Part print with two shaded views. Sizes in mm from the minimum x, y, z corner. A direction names the side the tool comes from. Coordinates: 2 decimals unless noted, no trailing zeros. Loops run counter-clockwise (first coordinate to the right, second up) from the corner with the lowest first, then second, coordinate; pieces in that order, holes last. Notation, with made-up numbers: (31.25, -35) -> (70.25, -35) arc R12 ccw to (70.25, -15) -> close; hole circle Ø8 at (64.25, 37.5). An arc over 180 degrees is marked (long way). Write each question's results on one line, items separated by ' | '.
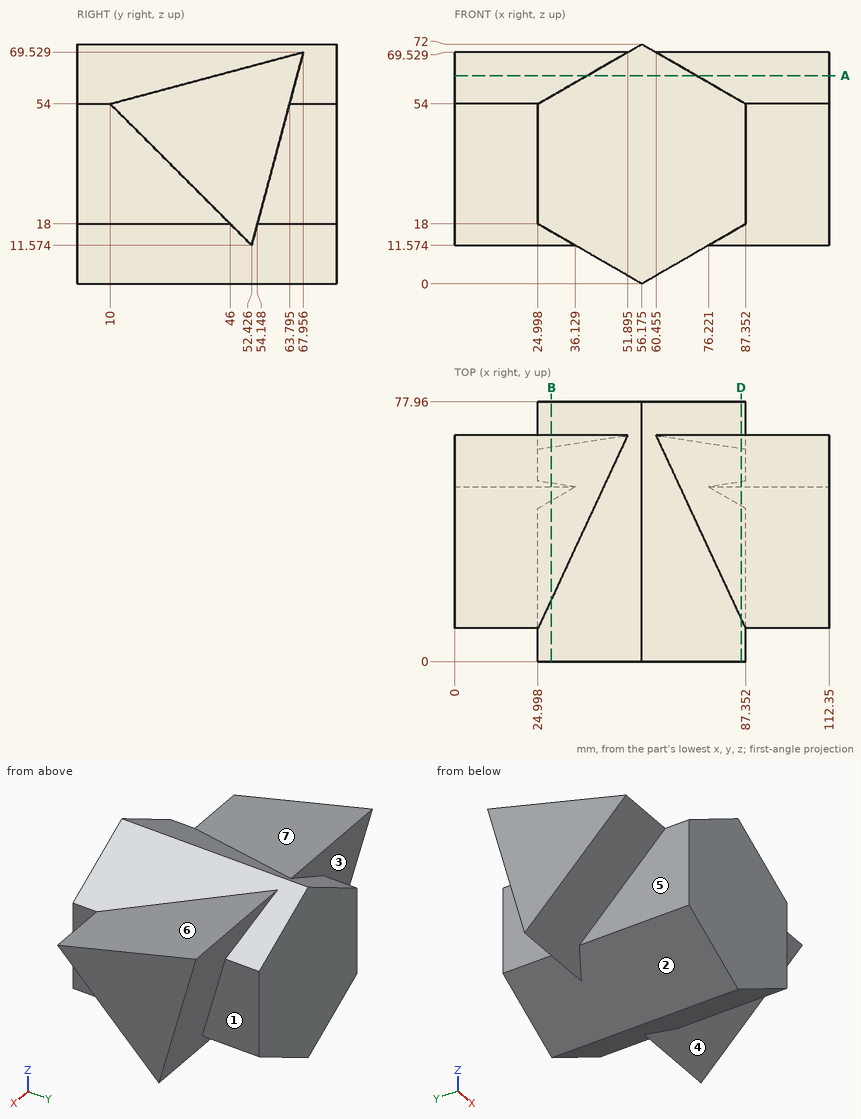
Q1. Pull direction X, two halves, no side cores. Call the marked faces 1, 2 and 3: +X half, -X half, draft (parallel to the pull), parting line (faces both ways), or undercut.
Results are:
face 1: +X half | face 2: -X half | face 3: draft
Q2. Which spindle directions (+Z, -Z, +X, -X, +Y, -Y) get a long thin tool onto all of the face, cutting with end or side? Do the marked faces 4, 5, 6 and 7. Say none if no direction does.
Results are:
face 4: -Z, +X, -Y | face 5: -Z, -X, -Y | face 6: +Z, +X, -Y | face 7: +Z, -X, -Y
Q3. Drop flat-ended pins along their axis: pin 1 (1.5 mm diameter, centred on x = 17.5, z = 31.5, fed in from -Y); pin 2 (1.5 mm diameter, centred on x = 17, y = 31.5, fed in from -Z); pin 3 (1.5 mm diameter, centred on x = 85, y = 28.5, fed in from -Z); pin 4 (1.5 mm diameter, centred on y = 46.5, z = 32.5, fed in from -X). Give the stop position or say it passes through.
Results are:
pin 1: y = 31.75 | pin 2: z = 31.75 | pin 3: z = 16.21 | pin 4: x = 0
Q4. Cut at D-D on x = 86. Write the cut outline in (y, z) (1 decimal).
Results are:
outline: (0, 17.2) -> (46.8, 17.2) -> (52.4, 11.6) -> (53.9, 17.2) -> (78, 17.2) -> (78, 54.8) -> (64, 54.8) -> (68, 69.5) -> (12.9, 54.8) -> (0, 54.8) -> close
Q5. Cut at A-A on z = 62.5. Write the cut outline in (x, y), and give its area (3 significant figures).
Results are:
outline: (0, 41.72) -> (39.72, 41.72) -> (39.72, 0) -> (72.63, 0) -> (72.63, 41.72) -> (112.35, 41.72) -> (112.35, 66.07) -> (72.63, 66.07) -> (72.63, 77.96) -> (39.72, 77.96) -> (39.72, 66.07) -> (0, 66.07) -> close | area: 4,500 mm^2
Q6. Cut at B-B on x = 29. Write the cut outline in (y, z) (1 decimal).
Results are:
outline: (0, 15.7) -> (48.3, 15.7) -> (52.4, 11.6) -> (53.5, 15.7) -> (78, 15.7) -> (78, 56.3) -> (64.4, 56.3) -> (68, 69.5) -> (18.6, 56.3) -> (0, 56.3) -> close
Q7. Wall check: L1, parallel to X at y = 58.5, z = 19; L2, parallel to Z at x = 59.5, y = 6; L3, parallel to Z at x = 78.5, y = 6. Give the ranges that are in metal, low to high. Write a range as from..to.
Results are:
L1: 25..87.35 | L2: 1.92..70.08 | L3: 12.89..59.11
